Input: part model. Units: mm. Frame: model coordinates. A direction names the side the tool comes from. Round coordinates to 2 decimals unless told otherwise and drop trailing zeros. Loops run counter-clockwise (first coordinate to the right, second up) from the corner with the lowest first, then second, coordinate; pieces in that order, holes last.
(1) Line query: line 1 (X direction, y = 5, z = -15); line 2 (X direction, y = 5.5, z = -18.8); line 3 (Z direction, x = -17, y = 8.25). Output: solid intervals per line, ascending.
(2) Cut plane D-D, the plane y = 5.5. Give the number of separate pieces and of enclosed holes in the cut face, and give its area (3 significant figures).
(3) Cut plane A-A, the plane z = 0. Output: boundary loops of the cut face in (x, y), and give its area (3 significant figures).
(4) Access query for faces 1 (the face through (-15, 6, 17)), 2 (the face through (-19.732, 7.675, -15.479)), 3 (the face through (17.7, 8.1, 14)). Directions: +Z, -Z, +X, -X, +Y, -Y. A direction counts if a zero-diameter tool reaches every point of the face in a straight line with its end or side. Return the directions, or none.
(5) Cut plane C-C, the plane z = 16. Output: boundary loops of the cut face in (x, y), and give its area (3 significant figures).
(6) First-contact query: pin 1 Ø3 at (x, z) = (12, 0.5) entering from +Y. Flat tip, straight axial feed; report the tip coordinate or a pass-through.
(7) Draft query along Y for faces 4 (the face through (-0.3, 2.8, 20)), 5 (the face through (16, 5, -15)), 6 (the face through (19.768, 3.345, 15.479)), 7 (the face through (22.2, 10, -0.3)). Return one class per face: released by +Y, released by -Y, zero draft, split by the parting line, or undercut.
(8) Cut plane B-B, the plane x = 0. Output: boundary loops of the cut face in (y, z), and give its area (3 significant figures).
from build123d import *

# Parameters (mm, degrees)
SKETCH1_W            = 50
SKETCH1_H            = 40
BOSS_EXTRUDE1_DEPTH  = 3
SKETCH2_R            = 12
CUT_EXTRUDE1_DEPTH   = 33.155870382
SKETCH3_W            = 3
SKETCH3_H            = 40
BOSS_EXTRUDE2_DEPTH  = 7
SKETCH4_W            = 7
SKETCH4_H            = 7
BOSS_EXTRUDE3_DEPTH  = 6
SKETCH5_R            = 1.75
CUT_EXTRUDE2_DEPTH   = 49.218253805
CUT_EXTRUDE3_DEPTH   = 3
MIRROR3_COPY_1_DEPTH = 3


with BuildPart() as part:
    # Sketch1 → Boss-Extrude1 (new body)
    with BuildSketch(Plane(origin=(0, 0, 0), x_dir=(1, 0, 0), z_dir=(0, 1, 0))):
        Rectangle(SKETCH1_W, SKETCH1_H)
    extrude(amount=BOSS_EXTRUDE1_DEPTH)

    # Sketch2 → Cut-Extrude1 (cut, through all)
    with BuildSketch(Plane(origin=(0, 3, 0), x_dir=(1, 0, 0), z_dir=(0, 1, 0))):
        with Locations(Location((0, 0, 0), (0, 0, 270))):
            Circle(SKETCH2_R)
    extrude(amount=-CUT_EXTRUDE1_DEPTH, mode=Mode.SUBTRACT)

    # Sketch3 → Boss-Extrude2 (add)
    with BuildSketch(Plane(origin=(0, 3, 0), x_dir=(1, 0, 0), z_dir=(0, 1, 0))):
        with Locations((-23.5, 0)):
            Rectangle(SKETCH3_W, SKETCH3_H)
        with Locations((23.5, 0)):
            Rectangle(SKETCH3_W, SKETCH3_H)
    extrude(amount=BOSS_EXTRUDE2_DEPTH)

    # Sketch4 → Boss-Extrude3 (add)
    with BuildSketch(Plane.XY.offset(20)):
        with Locations((-18.5, 6.5)):
            Rectangle(SKETCH4_W, SKETCH4_H)
        with Locations((18.5, 6.5)):
            Rectangle(SKETCH4_W, SKETCH4_H)
    boss_extrude3 = extrude(amount=-BOSS_EXTRUDE3_DEPTH)

    # Sketch5 → Cut-Extrude2 (cut, through all)
    with BuildSketch(Plane.XY.offset(20)):
        with Locations((-18.5, 5.5)):
            Circle(SKETCH5_R)
        with Locations((18.5, 5.5)):
            Circle(SKETCH5_R)
    cut_extrude2 = extrude(amount=-CUT_EXTRUDE2_DEPTH, mode=Mode.SUBTRACT)

    # Mirror1: Boss-Extrude3, Cut-Extrude2 across plane
    add(boss_extrude3.mirror(Plane.XY))
    add(cut_extrude2.mirror(Plane.XY), mode=Mode.SUBTRACT)

    # Sketch6 → Cut-Extrude3 (cut)
    with BuildSketch(Plane.XY.offset(-14)):
        Polygon((-18.5, 2.613248654), (-16, 4.056624327), (-16, 6.943375673), (-18.5, 8.386751346), (-21, 6.943375673), (-21, 4.056624327), align=None)
    cut_extrude3 = extrude(amount=-CUT_EXTRUDE3_DEPTH, mode=Mode.SUBTRACT)

    # Mirror2: Cut-Extrude3 across plane
    add(cut_extrude3.mirror(Plane(origin=(0, 0, 0), x_dir=(0, 0, 1), z_dir=(1, 0, 0))), mode=Mode.SUBTRACT)

    # Mirror3: Cut-Extrude3 across plane
    add(cut_extrude3.mirror(Plane.XY), mode=Mode.SUBTRACT)

    # Mirror3 copy 1 sketch → Mirror3 copy 1 (cut)
    with BuildSketch(Plane(origin=(0, 0, 14), x_dir=(-1, 0, 0), z_dir=(0, 0, -1))):
        Polygon((-18.5, 2.613248654), (-16, 4.056624327), (-16, 6.943375673), (-18.5, 8.386751346), (-21, 6.943375673), (-21, 4.056624327), align=None)
    extrude(amount=-MIRROR3_COPY_1_DEPTH, mode=Mode.SUBTRACT)


solid = part.part
Reported:
1. line 1: x = -25 to -21, -16 to -15, 15 to 16, 21 to 25
1. line 2: x = -25 to -20.25, -16.75 to -15, 15 to 16.75, 20.25 to 25
1. line 3: z = -20 to -14, 14 to 20
2. separate pieces: 6
2. enclosed holes: 0
2. area: 306 mm2
3. outline: (-25, 0) - (-12, 0) - (-12, 3) - (-22, 3) - (-22, 10) - (-25, 10) - close; (12, 0) - (25, 0) - (25, 10) - (22, 10) - (22, 3) - (12, 3) - close
3. area: 120 mm2
4. face 1: +Z, -Z, +Y
4. face 2: none
4. face 3: +Y
5. outline: (-25, 0) - (25, 0) - (25, 10) - (15, 10) - (15, 3) - (-15, 3) - (-15, 10) - (-25, 10) - close; hole (-21, 4.06) - (-18.5, 2.61) - (-16, 4.06) - (-16, 6.94) - (-18.5, 8.39) - (-21, 6.94) - close; hole (16, 4.06) - (18.5, 2.61) - (21, 4.06) - (21, 6.94) - (18.5, 8.39) - (16, 6.94) - close
5. area: 247 mm2
6. pin 1: stops at y = 3
7. face 4: zero draft
7. face 5: undercut
7. face 6: undercut
7. face 7: released by +Y
8. outline: (0, -20) - (3, -20) - (3, -12) - (0, -12) - close; (0, 12) - (3, 12) - (3, 20) - (0, 20) - close
8. area: 48.0 mm2
